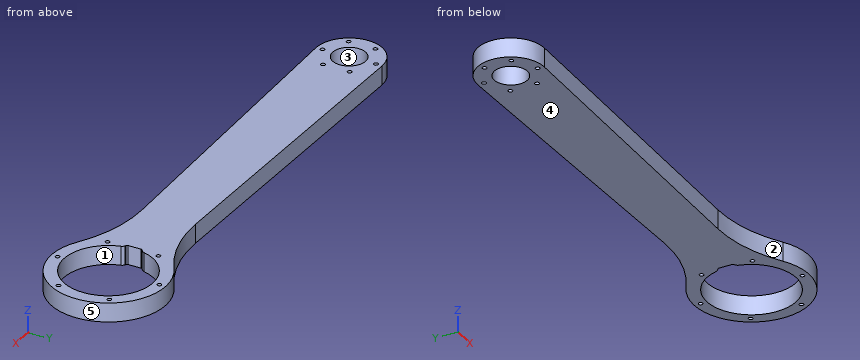
from build123d import *

# Parameters (mm, degrees)
SKETCH_1_R      = 1.65
SKETCH_1_R_2    = 13
SKETCH_1_R_3    = 1.7
EXTRUDE_1_DEPTH = 15


with BuildPart() as part:
    # 草图1 → 凸台-拉伸1 (new body)
    with BuildSketch(Plane.XY):
        with BuildLine():
            Line((-85.245113537, 20.900392521), (-339.479111624, 25.994781694))
            ThreePointArc((-339.479111624, 25.994781694), (-366, 0), (-339.479111624, -25.994781694))
            Line((-339.479111624, -25.994781694), (-85.245113537, -20.900392521))
            ThreePointArc((-85.245113537, -20.900392521), (-53.416829007, -24.942544633), (-24.108780491, -37.996930182))
            ThreePointArc((-24.108780491, -37.996930182), (45, 0), (-24.108780491, 37.996930182))
            ThreePointArc((-24.108780491, 37.996930182), (-53.416829007, 24.942544633), (-85.245113537, 20.900392521))
        make_face()
        with Locations((0, 40)):
            Circle(SKETCH_1_R, mode=Mode.SUBTRACT)
        with Locations((34.641016151, 20)):
            Circle(SKETCH_1_R, mode=Mode.SUBTRACT)
        with Locations((34.641016151, -20)):
            Circle(SKETCH_1_R, mode=Mode.SUBTRACT)
        with Locations((0, -40)):
            Circle(SKETCH_1_R, mode=Mode.SUBTRACT)
        with Locations((-34.641016151, 20)):
            Circle(SKETCH_1_R, mode=Mode.SUBTRACT)
        with Locations((-34.641016151, -20)):
            Circle(SKETCH_1_R, mode=Mode.SUBTRACT)
        with Locations((-340, 0)):
            Circle(SKETCH_1_R_2, mode=Mode.SUBTRACT)
        with Locations((-340, 21)):
            Circle(SKETCH_1_R_3, mode=Mode.SUBTRACT)
        with Locations((-358.186533479, 10.5)):
            Circle(SKETCH_1_R_3, mode=Mode.SUBTRACT)
        with Locations((-358.186533479, -10.5)):
            Circle(SKETCH_1_R_3, mode=Mode.SUBTRACT)
        with Locations((-340, -21)):
            Circle(SKETCH_1_R_3, mode=Mode.SUBTRACT)
        with Locations((-321.813466521, -10.5)):
            Circle(SKETCH_1_R_3, mode=Mode.SUBTRACT)
        with Locations((-321.813466521, 10.5)):
            Circle(SKETCH_1_R_3, mode=Mode.SUBTRACT)
        with BuildLine():
            Line((-35.500051413, 6.790401018), (-36.237951224, 6.373427606))
            ThreePointArc((-36.237951224, 6.373427606), (-36.795555255, 5.823507629), (-37, 5.067507244))
            Line((-37, 5.067507244), (-37, -5.067507244))
            ThreePointArc((-37, -5.067507244), (-36.795555255, -5.823507629), (-36.237951224, -6.373427606))
            Line((-36.237951224, -6.373427606), (-35.500051413, -6.790401018))
            ThreePointArc((-35.500051413, -6.790401018), (-34.451431588, -7.698788042), (-33.838125094, -8.943225935))
            ThreePointArc((-33.838125094, -8.943225935), (35, 0), (-33.838125094, 8.943225935))
            ThreePointArc((-33.838125094, 8.943225935), (-34.451431588, 7.698788042), (-35.500051413, 6.790401018))
        make_face(mode=Mode.SUBTRACT)
    extrude(amount=EXTRUDE_1_DEPTH)


solid = part.part
Work out the finished part from the listing and answer in its coordinate system (mm). Face numbers are marked on the shaded views. A direction names the side the tool comes from. Give positions to 0.01 mm unless a question says otherwise; leave off trailing zeros. Order: outer loops, then holes, each group sorted by start corner. A loop starts at its lowest first (then second) coordinate and runs counter-clockwise, first axis right, second up. Notation, with made-up numbers: (55, 40) - (81, 40) arc R14 cw to (81, 57) - close; hole circle Ø7 at (68, -8.75). An arc over 180 degrees is marked (long way). Answer as CSV lines item,"result". Start each with the question number.
Q1. The mould has two halves that part along Y. Classify the marked faces 3, 4 and 5: +Y half, -Y half, draft (parallel to the pull), parting line (faces both ways), or undercut.
Q2. Given pin 1 Ø2.5 at (x, y) = (34.64, -20) entering from -Z; pin 2 Ø8 at (y, z) = (-2, 7.5) entering from +X; pin 3 Ø1 at (y, z) = (-31.5, 9) entering from +X; pin 4 Ø8 at (x, z) = (-74, 13) entering from -Y, each flat-ended and moving along its own axis, determine where each tip first touches the part or whether it passes through.
Q3. The part is cut by section C-C (x = -200). Write down the section's boundary in (y, z).
Q4. The part is cut by section B-B (x = -290). Write down the section's boundary in (y, z), then the cut area to 3 significant figures.
Q5. Find the intervals of material crossed by L1, parallel to Y at x = 0, z = 11.75; L2, parallel to X at y = -6, z = 12.5; L3, parallel to X at y = -1.5, z = 9.25 (3 decimals), in increasing order. Write a range as [from, to].
Q6. For the marked faces 1 and 2, determine the directions among +Z, -Z, +X, -X, +Y, -Y from which every point of the face is accessible in a straight line to the end or side of a thin tool.
Q7. The part is cut by section A-A (z = 6.75). Give the number of separate pieces and of enclosed holes in the cut face, then the cut area to 3 significant figures.
Check result:
1,face 3,"undercut"
1,face 4,"draft"
1,face 5,"parting line"
2,pin 1,"passes through"
2,pin 2,"stops at x = 45"
2,pin 3,"stops at x = 32.62"
2,pin 4,"stops at y = -21.65"
3,outline,"(-23.2, 0) - (23.2, 0) - (23.2, 15) - (-23.2, 15) - close"
4,outline,"(-25, 0) - (25, 0) - (25, 15) - (-25, 15) - close"
4,area,"750 mm²"
5,L1,"y = [-45, -41.65], [-38.35, -35], [35, 38.35], [41.65, 45]"
5,L2,"x = [-365.3, -351.53], [-328.47, -36.67], [34.48, 44.6]"
5,L3,"x = [-365.957, -352.913], [-327.087, -37], [34.968, 44.975]"
6,face 1,"+Z, -Z"
6,face 2,"+Z, -Z, -Y"
7,separate pieces,"1"
7,enclosed holes,"14"
7,area,"16,900 mm²"
